Verification items for this drawing (mm, ordinates from the low corner). A direction names the side the tool comes from. Round coordinates to 2 decimals unless told otherwise and drop trailing zeros. Loops run counter-clockwise (first coordinate to the right, second up) from the corner with the lowest first, then second, coordinate; pieces in that order, holes last. Notation, with made-up numbers: M 52,21 L 92,21 A22 ccw 92,57 Z; hole C -12,60.5 d9. An arc over 180 degrees is marked long. One line per item, written item: value.
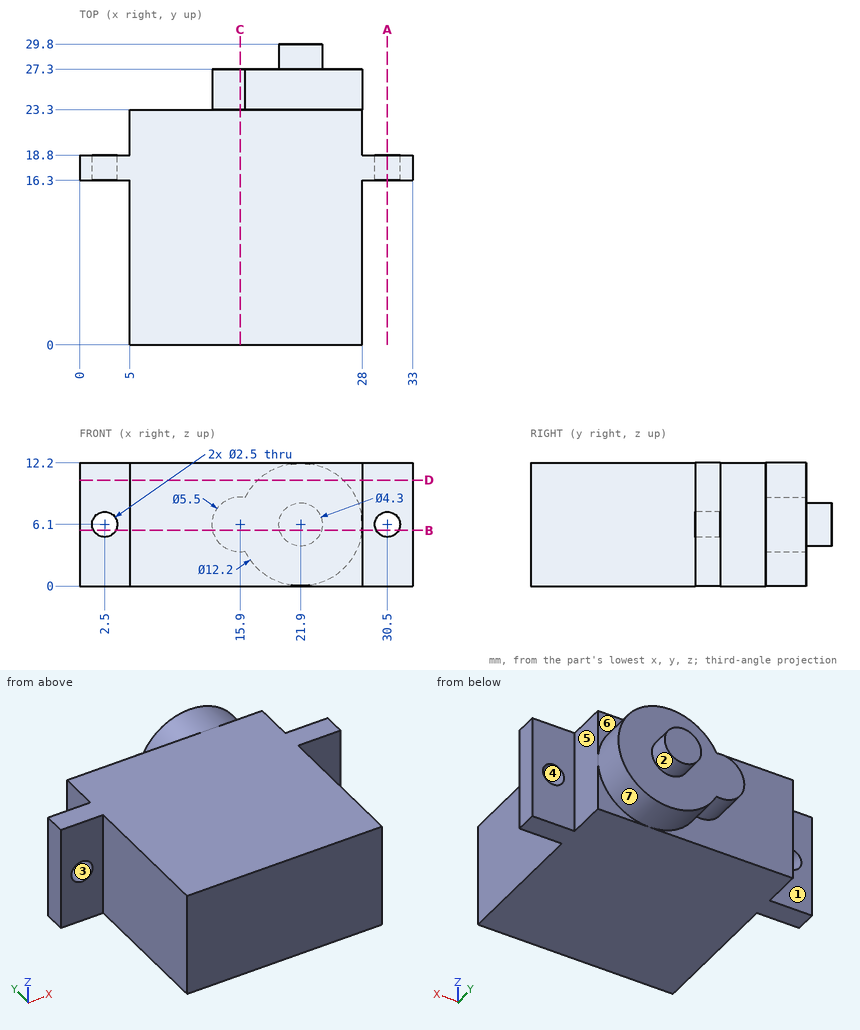
(1) Sectioned sample at A-A on x = 30.5. Enter the section's corners in (y, z).
Completed:
outline: M 16.3,0 L 18.8,0 L 18.8,4.85 L 16.3,4.85 Z; M 16.3,7.35 L 18.8,7.35 L 18.8,12.2 L 16.3,12.2 Z
(2) Thickness scan on L1, parallel to X at y = 18.3, z = 6.1; L2, parallel to Z at x = 30.5, y = 17.55; L3, parallel to X at y = 16.25, z = 5. Record the ranges inside material, lowest first. Write a range as from..to.
Completed:
L1: x = 0..1.25, 3.75..29.25, 31.75..33
L2: z = 0..4.85, 7.35..12.2
L3: x = 5..28
(3) Mould release check, pull along X, two halves, no side actions. Record for the marked faces 1, 2, 3 and 4: +X half, -X half, draft (parallel to the pull), parting line (faces both ways), or undercut.
Completed:
face 1: draft
face 2: parting line
face 3: undercut
face 4: undercut
(4) Sectioned sample at C-C on x = 15.9. Enter the section's corners in (y, z).
Completed:
outline: M 0,0 L 23.3,0 L 23.3,3.35 L 27.3,3.35 L 27.3,8.85 L 23.3,8.85 L 23.3,12.2 L 0,12.2 Z
(5) Tool access check on the marked faces 5, 6 and 7. Record the directions out of +Z, -Z, +X, -X, +Y, -Y that give a thin tool (end or side, any length) a straight path to the whole face; none if there is none.
Completed:
face 5: +Z, -Z, +X, +Y
face 6: +Z, +X, +Y
face 7: +Y
(6) Sectioned sample at D-D on z = 10.5. Enter the section's corners in (x, y), and give its area (3 significant figures).
Completed:
outline: M 0,16.3 L 5,16.3 L 5,0 L 28,0 L 28,16.3 L 33,16.3 L 33,18.8 L 28,18.8 L 28,23.3 L 26.12,23.3 L 26.12,27.3 L 17.68,27.3 L 17.68,23.3 L 5,23.3 L 5,18.8 L 0,18.8 Z
area: 595 mm^2
(7) Sectioned sample at B-B on z = 5.5. Count the separate pieces of the cut face and the enclosed holes in it, and give its area (3 significant figures).
Completed:
separate pieces: 3
enclosed holes: 0
area: 619 mm^2
(8) Depth check by flat-ended pin: pin 1 Ø1.8 at (x, z) = (24, 9.5) entering from +Y; pin 2 Ø3.5 at (y, z) = (7, 8.5) entering from +X; pin 3 Ø3.5 at (y, z) = (8, 6.5) entering from -X; pin 4 Ø2 at (x, z) = (30.5, 6.1) entering from +Y. Enter the tip coordinate at first touch or a pass-through.
Completed:
pin 1: stops at y = 27.3
pin 2: stops at x = 28
pin 3: stops at x = 5
pin 4: passes through
